Build history of the part. All positions in model axes, mm. Face numbers are marked on the shaded views. A direction names the side the tool comes from. Round coordinates to 2 decimals unless told otherwise and drop trailing zeros. Write each loop counter-clockwise with the first axis right and the second up, starting at its lowest first coordinate (ties: lowest second). Pieces come first, ordered by that corner, then holes.
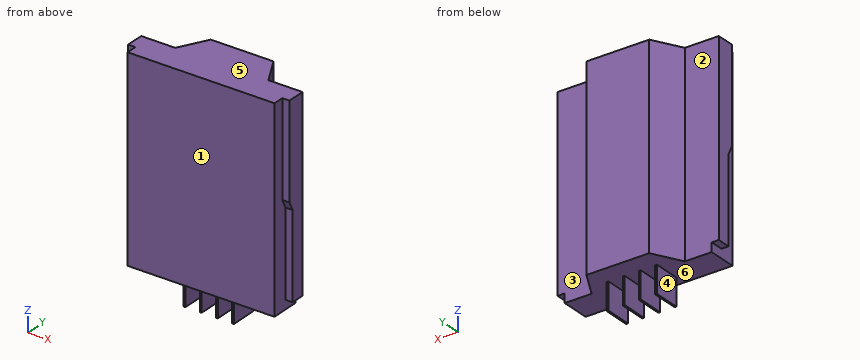
from build123d import *

# Parameters (mm, degrees)
PAD_DEPTH       = 110
POCKET_DEPTH    = 4
POCKET002_DEPTH = 4
SKETCH003_W     = 1
SKETCH003_H     = 15
PAD001_DEPTH    = 15


with BuildPart() as part:
    # Sketch → Pad (new body)
    with BuildSketch(Plane.XY):
        Polygon((-17.5, 25.7), (17.5, 25.7), (26, 10), (45, 10), (45, 0), (41, 0), (41, -6), (-41, -6), (-41, 0), (-45, 0), (-45, 10), (-26, 10), align=None)
    extrude(amount=PAD_DEPTH)

    # Sketch001 → Pocket (cut)
    with BuildSketch(Plane.YZ.offset(-45)):
        Polygon((2.5, 5), (10, 5), (10, 0), (0, 0), (0, 57.5), (2.5, 52.5), align=None)
    extrude(amount=POCKET_DEPTH, mode=Mode.SUBTRACT)

    # Sketch002 → Pocket002 (cut)
    with BuildSketch(Plane.YZ.offset(45)):
        Polygon((2.5, 5), (10, 5), (10, 0), (0, 0), (0, 57.5), (2.5, 52.5), align=None)
    extrude(amount=-POCKET002_DEPTH, mode=Mode.SUBTRACT)

    # Sketch003 → Pad001 (join)
    with BuildSketch(Plane.XY):
        with Locations((-13.5, 7.5)):
            Rectangle(SKETCH003_W, SKETCH003_H)
        with Locations((-4.5, 7.5)):
            Rectangle(SKETCH003_W, SKETCH003_H)
        with Locations((4.5, 7.5)):
            Rectangle(SKETCH003_W, SKETCH003_H)
        with Locations((13.5, 7.5)):
            Rectangle(SKETCH003_W, SKETCH003_H)
    extrude(amount=-PAD001_DEPTH)


solid = part.part
1) Slice it at B-B (z = 62.5). Write the cut outline in (x, y), plus the area to 3 significant figures.
Results:
outline: (-45, 0) - (-41, 0) - (-41, -6) - (41, -6) - (41, 0) - (45, 0) - (45, 10) - (26, 10) - (17.5, 25.7) - (-17.5, 25.7) - (-26, 10) - (-45, 10) - close
area: 2,070 mm2
2) Slice it at A-A (z = -4). Write the cut outline in (x, y), plus the area to 3 significant figures.
Results:
outline: (-14, 0) - (-13, 0) - (-13, 15) - (-14, 15) - close; (-5, 0) - (-4, 0) - (-4, 15) - (-5, 15) - close; (4, 0) - (5, 0) - (5, 15) - (4, 15) - close; (13, 0) - (14, 0) - (14, 15) - (13, 15) - close
area: 60.0 mm2
3) Mould opens along X. For the marked faces 4, 5 and 6 say: released by +X, released by -X, zero draft, split by the parting line, or undercut.
Results:
face 4: released by -X
face 5: zero draft
face 6: undercut
4) Slice it at D-D (x = -9). Write the cut outline in (y, z).
Results:
outline: (-6, 0) - (25.7, 0) - (25.7, 110) - (-6, 110) - close
5) Pin check, flat tips, straight feed: pin 1 Ø0.5 at (x, z) = (-4.5, -9) entering from +Y; pin 2 Ø0.8 at (x, z) = (-13.5, -5) entering from -Y; pin 3 Ø4.5 at (x, z) = (43.5, 24.5) entering from -Y. Stop position of each tip, or through.
Results:
pin 1: stops at y = 15
pin 2: stops at y = 0
pin 3: stops at y = 2.5
6) Wall check: L1, parallel to Z at x = 19.5, y = 8.5; L2, parallel to Y at x = -37.5, z = 39.5; L3, parallel to Y at x = -19, z = 19. Give the ranges that are in metal, low to high.
Results:
L1: z = 0 to 110
L2: y = -6 to 10
L3: y = -6 to 22.93
7) Slice it at C-C (y = 6). Write the cut outline in (x, z).
Results:
outline: (-45, 5) - (-41, 5) - (-41, 0) - (-14, 0) - (-14, -15) - (-13, -15) - (-13, 0) - (-5, 0) - (-5, -15) - (-4, -15) - (-4, 0) - (4, 0) - (4, -15) - (5, -15) - (5, 0) - (13, 0) - (13, -15) - (14, -15) - (14, 0) - (41, 0) - (41, 5) - (45, 5) - (45, 110) - (-45, 110) - close
8) Which spindle directions (+Z, -Z, +X, -X, +Y, -Y) get a long thin tool onto all of the face, cutting with end or side? Do the marked faces 1, 2 and 3. Say none if no direction does.
Results:
face 1: +Z, -Z, +X, -X, -Y
face 2: +Z, -Z, -X, +Y
face 3: +Z, -Z, +X, +Y
